Design review of the part built by this model. Coordinates are the model's own, in mm. Give positions to 0.01 mm unless a question says otherwise; leave off trailing zeros. Order: outer loops, then holes, each group sorted by start corner. A loop starts at its lowest first (then second) coordinate and runs counter-clockwise, first axis right, second up. Notation, with made-up numbers: (29, -11.75) -> (47, -11.75) arc R14 ccw to (47, -3.75) -> close; hole circle Ø2 at (10, 27.25). An arc over 180 degrees is marked (long way). Use a Markdown table: item, result. Add a question column.
```python
from build123d import *

# Parameters (mm, degrees)
SKETCH1_W           = 32.9
SKETCH1_H           = 140
BOSS_EXTRUDE1_DEPTH = 20
SKETCH3_R           = 6
CUT_EXTRUDE1_DEPTH  = 33.9
FILLET1_R           = 1


with BuildPart() as part:
    # Sketch1 → Boss-Extrude1 (new body)
    with BuildSketch(Plane.XY):
        Rectangle(SKETCH1_W, SKETCH1_H)
    extrude(amount=BOSS_EXTRUDE1_DEPTH)

    # Sketch3 → Cut-Extrude1 (cut, through all)
    with BuildSketch(Plane(origin=(16.45, 0, 0), x_dir=(0, 0, -1), z_dir=(1, 0, 0))):
        with Locations((-10, 60)):
            Circle(SKETCH3_R)
        with Locations((-10, -60)):
            Circle(SKETCH3_R)
    extrude(amount=-CUT_EXTRUDE1_DEPTH, mode=Mode.SUBTRACT)

    # Fillet1
    fillet1_edges = [part.edges().sort_by_distance(p)[0] for p in [
        (-16.45, 0, 20),
        (0, -70, 20),
        (16.45, 0, 20),
        (0, -70, 0),
        (-16.45, 0, 0),
        (0, 70, 0),
        (16.45, 0, 0),
        (0, 70, 20),
        (16.45, -70, 10),
        (-16.45, -70, 10),
        (-16.45, 70, 10),
        (16.45, 70, 10),
    ]]
    fillet(fillet1_edges, radius=FILLET1_R)


solid = part.part
```
1) Add section C-C (z = 10). Give the boundary of the cut face in (x, y).
2) Insertion check: pin 1 (7 mm diameter, centred on y = 60, z = 10, fed in from -X). The pin has a flat end and moves straight along its axis. Give the tip position at first contact, or say it passes through.
3) Add section B-B (y = 60). Give the boundary of the cut face in (x, z).
4) For L1, parallel to Y at x = 1.5, z = 10; L2, parallel to Y at x = 14.5, z = 6, list the stretches that pass through material, from the lowest coordinate up. Write a range as [from, to].
5) Add section A-A (x = 4.5). Give the boundary of the cut face in (y, z), then the cut area to 3 significant figures.
6) The part is to be moulded in two halves that separate along Z. For faces 1 (the flat face through (0, 1, 0)), 2 (the flat face through (0, 1, 20)), 3 (the cylindrical face through (0.23, 57.7, 4.46)), say which applies: +Z half, -Z half, draft (parallel to the pull), parting line (faces both ways), or undercut.
Worked answers:
| question | item | result |
|---|---|---|
| 1 | outline | (-16.45, -69) arc R1 ccw to (-15.45, -70) -> (15.45, -70) arc R1 ccw to (16.45, -69) -> (16.45, -66) -> (-16.45, -66) -> close; (-16.45, -54) -> (16.45, -54) -> (16.45, 54) -> (-16.45, 54) -> close; (-16.45, 66) -> (16.45, 66) -> (16.45, 69) arc R1 ccw to (15.45, 70) -> (-15.45, 70) arc R1 ccw to (-16.45, 69) -> close |
| 2 | pin 1 | through |
| 3 | outline | (-16.45, 1) arc R1 ccw to (-15.45, 0) -> (15.45, 0) arc R1 ccw to (16.45, 1) -> (16.45, 4) -> (-16.45, 4) -> close; (-16.45, 16) -> (16.45, 16) -> (16.45, 19) arc R1 ccw to (15.45, 20) -> (-15.45, 20) arc R1 ccw to (-16.45, 19) -> close |
| 4 | L1 | [-70, -66], [-54, 54], [66, 70] |
| 4 | L2 | [-70, -64.47], [-55.53, 55.53], [64.47, 70] |
| 5 | outline | (-70, 1) arc R1 ccw to (-69, 0) -> (69, 0) arc R1 ccw to (70, 1) -> (70, 19) arc R1 ccw to (69, 20) -> (-69, 20) arc R1 ccw to (-70, 19) -> close; hole circle Ø12 at (-60, 10); hole circle Ø12 at (60, 10) |
| 5 | area | 2,570 mm^2 |
| 6 | face 1 | -Z half |
| 6 | face 2 | +Z half |
| 6 | face 3 | undercut |
